Work out the finished part from the listing and answer in its coordinate system (mm). Round coordinates to 2 decimals unless told otherwise and drop trailing zeros. Order: outer loops, then holes, each group sorted by start corner. A loop starts at its lowest first (then second) coordinate and runs counter-clockwise, first axis right, second up. Notation, with made-up numbers: (30, 25) - (51, 25) arc R9 ccw to (51, 42) - close; hole circle Ø4 at (56.25, 5). An arc over 180 degrees is marked (long way). One line per question, with ' | ' between items. Start each with the question number.
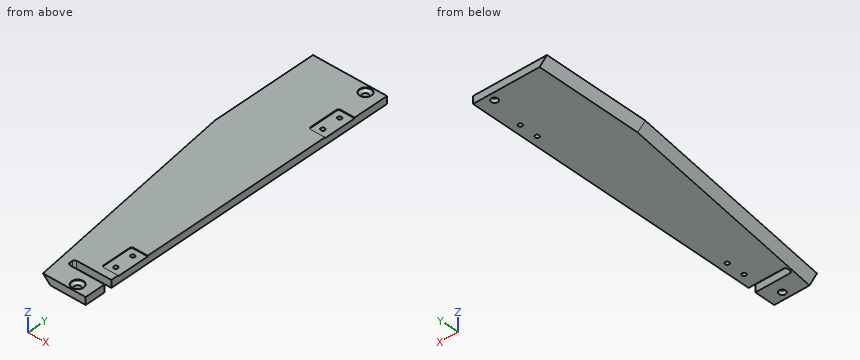
from build123d import *

# Parameters (mm, degrees)
BOSS_EXTRUDE1_DEPTH                          = 10
CHAMFER1_SIZE                                = 10
CSK_FOR_M8_HEX_SOCKET_COUNTERSUNK_HE_2_COUNT = 2
CSK_FOR_M8_HEX_SOCKET_COUNTERSUNK_HE_2_PITCH = 427
CUT_EXTRUDE1_DEPTH                           = 30
CUT_EXTRUDE2_DEPTH                           = 1
SKETCH6_R                                    = 2.75
CUT_EXTRUDE3_DEPTH                           = 459.137533935


with BuildPart() as part:
    # Sketch1 → Boss-Extrude1 (new body)
    with BuildSketch(Plane.XY):
        Polygon((0, 0), (-100, 0), (-100, -146), (-57.697208755, -447), (0, -447), align=None)
    extrude(amount=BOSS_EXTRUDE1_DEPTH)

    # Chamfer1
    chamfer1_edges = [part.edges().sort_by_distance(p)[0] for p in [
        (-78.848604377, -296.5, 0),
        (-100, -73, 0),
    ]]
    chamfer(chamfer1_edges, length=CHAMFER1_SIZE - 0.0001)  # a hair under: the kernel refuses the full size

    # Sketch3 → CSK for M8 Hex Socket Countersunk Head Screw1 (revolve, cut)
    with BuildSketch(Plane(origin=(-20, -10, 10), x_dir=(0, -1, 0), z_dir=(1, 0, 0))):
        Polygon((0, 0), (0, 10), (4.5, 10), (4.5, 4.5), (8, 1), (8, 0), align=None)
    csk_for_m8_hex_socket_countersunk_head_s = revolve(axis=Axis((-20, -10, 16.35), (0, 0, -1)), mode=Mode.SUBTRACT)

    # CSK for M8 Hex Socket Countersunk He 2: CSK for M8 Hex Socket Countersunk Head Screw1 ×2
    with Locations(*[(0, -i * CSK_FOR_M8_HEX_SOCKET_COUNTERSUNK_HE_2_PITCH, 0) for i in range(1, CSK_FOR_M8_HEX_SOCKET_COUNTERSUNK_HE_2_COUNT)]):
        add(csk_for_m8_hex_socket_countersunk_head_s, mode=Mode.SUBTRACT)

    # Sketch4 → Cut-Extrude1 (cut)
    with BuildSketch(Plane.XY.offset(10)):
        with BuildLine():
            Line((0, -409), (-46.897208755, -409))
            ThreePointArc((-46.897208755, -409), (-49.018529098, -409.878679656), (-49.897208755, -412))
            Line((-49.897208755, -412), (-49.897208755, -416))
            ThreePointArc((-49.897208755, -416), (-49.018529098, -418.121320344), (-46.897208755, -419))
            Line((-46.897208755, -419), (0, -419))
            Line((0, -419), (0, -409))
        make_face()
    extrude(amount=-CUT_EXTRUDE1_DEPTH, mode=Mode.SUBTRACT)

    # Sketch5 → Cut-Extrude2 (cut)
    with BuildSketch(Plane.XY.offset(10)):
        with BuildLine():
            Line((-19, -48), (0, -48))
            Line((0, -48), (0, -92))
            Line((0, -92), (-19, -92))
            ThreePointArc((-19, -92), (-21.121320344, -91.121320344), (-22, -89))
            Line((-22, -89), (-22, -51))
            ThreePointArc((-22, -51), (-21.121320344, -48.878679656), (-19, -48))
        make_face()
        with BuildLine():
            Line((-19, -355), (0, -355))
            Line((0, -355), (0, -399))
            Line((0, -399), (-19, -399))
            ThreePointArc((-19, -399), (-21.121320344, -398.121320344), (-22, -396))
            Line((-22, -396), (-22, -358))
            ThreePointArc((-22, -358), (-21.121320344, -355.878679656), (-19, -355))
        make_face()
    extrude(amount=-CUT_EXTRUDE2_DEPTH, mode=Mode.SUBTRACT)

    # Sketch6 → Cut-Extrude3 (cut, through all)
    with BuildSketch(Plane.XY.offset(9)):
        with Locations((-11.5, -57.5)):
            Circle(SKETCH6_R)
        with Locations((-11.5, -82.5)):
            Circle(SKETCH6_R)
        with Locations((-11.5, -364.5)):
            Circle(SKETCH6_R)
        with Locations((-11.5, -389.5)):
            Circle(SKETCH6_R)
    extrude(amount=-CUT_EXTRUDE3_DEPTH, mode=Mode.SUBTRACT)


solid = part.part
1) Section C-C on z = 3.25 is taken. Give the vertices of the cut face in (x, y), and give its area (3 significant figures).
2) Straight lines are drawn through the part: line 1 (Y direction, x = -11.5, z = 2.75); line 2 (Y direction, x = -20, z = 2.95); line 3 (Y direction, x = -15, z = 5.25). For each, find the intervals that lie inside material, in ascending order.
3) Section A-A on x = -33 is taken. Give the vertices of the cut face in (y, z).
4) Flat-ended cylindrical pins translate along their axes: pin 1 (2 mm diameter, centred on y = -188.5, z = 6, fed in from +X); pin 2 (4.5 mm diameter, centred on x = -11.5, y = -57.5, fed in from -Z); pin 3 (7 mm diameter, centred on x = -11.5, y = -364.5, fed in from +Z); pin 4 (2 mm diameter, centred on y = -413, z = 4, fed in from +X). Find the tip coordinate at first contact, or state that the pin passes through.
Recorded:
1) outline: (-93.25, -145.53) - (-50.88, -447) - (0, -447) - (0, -419) - (-46.9, -419) arc R3 cw to (-49.9, -416) - (-49.9, -412) arc R3 cw to (-46.9, -409) - (0, -409) - (0, 0) - (-93.25, 0) - close; hole circle Ø9 at (-20, -437); hole circle Ø9 at (-20, -10); hole circle Ø5.5 at (-11.5, -389.5); hole circle Ø5.5 at (-11.5, -364.5); hole circle Ø5.5 at (-11.5, -82.5); hole circle Ø5.5 at (-11.5, -57.5) | area: 34,600 mm²
2) line 1: y = -447 to -419, -409 to -392.25, -386.75 to -367.25, -361.75 to -85.25, -79.75 to -60.25, -54.75 to 0 | line 2: y = -447 to -441.5, -432.5 to -419, -409 to -14.5, -5.5 to 0 | line 3: y = -447 to -419, -409 to 0
3) outline: (-447, 0) - (-419, 0) - (-419, 10) - (-447, 10) - close; (-409, 0) - (0, 0) - (0, 10) - (-409, 10) - close
4) pin 1: stops at x = 0 | pin 2: passes through | pin 3: stops at z = 9 | pin 4: stops at x = -49.9
